Could you check a few things on this model? Use its own coordinates, in mm. A direction names the side the tool comes from. Coordinates: 2 decimals unless noted, no trailing zeros. Write each loop counter-clockwise with the first axis right and the second up, starting at its lowest first coordinate (ties: lowest second). Pieces come first, ordered by that corner, then holes. Notation, with made-up numbers: M 4.25,-16 L 45.25,-16 A10 ccw 45.25,-4 Z; hole C 30,47 d3. An arc over 180 degrees is marked long. Answer as CSV lines item,"result". Start each with the question number.
Item 1: If I drill on line 1 along Y through (x, z) = (52, 2.1); line 2 along Y through (x, z) = (54, 4.25); line 3 along Y through (x, z) = (6.5, 2), over which ranges is the centre line in solid material (lowest first)? Write a range as [from, to].
Item 2: Suppose I cut it at A-A, the plane y = 80. Write out the boundary of the cut face in (x, z).
Item 3: We'd pull the mould along X, two halves only. Please class faces 1 (the flat face through (30, 100, 10)), 2 (the cylindrical face through (29.133, 76.095, 10.274)), 3 (the cylindrical face through (49.253, 6.121, 8.549)), 4 (the flat face through (0, 42, 6)): +X half, -X half, draft (parallel to the pull), parting line (faces both ways), or undercut.
Item 4: I'm going to push flat-ended pins straight in: P1, Ø5, axis at x = 8.5, y = 6, coming from the -Z side; P2, Ø14, axis at x = 43, y = 80, coming from the -Z side; P3, Ø7, axis at x = 27.5, z = 4, coming from the +Y side. Where does each tip first touch, or does it pass through?
Item 5: Suppose I cut it at B-B, the plane x = 30. Write out the boundary of the cut face in (y, z), and give its area (3 significant figures).
Item 6: Suppose I cut it at D-D, the plane z = 1. Write out the boundary of the cut face in (x, y), and give its area (3 significant figures).
Item 7: On a 3-axis mill with a long thin cutter (end or side, diameter ignored), from which of +Z, -Z, +X, -X, +Y, -Y can I reach the whole of each face in a straight line? I mean faces 5 (the cylindrical face through (53.328, 68.054, 5.916)), 6 (the cylindrical face through (57, 6, 2)), 7 (the flat face through (30, 86, 8.5)). Say none if no direction works.
Item 8: Suppose I cut it at C-C, the plane y = 6. Write out the boundary of the cut face in (x, z).
```python
from build123d import *

# Parameters (mm, degrees)
ESQUISSE2_W                                        = 60
ESQUISSE2_H                                        = 100
BOSS_EXTRU_1_DEPTH                                 = 12
ESQUISSE3_R                                        = 4
ENL_V_MAT_EXTRU_1_DEPTH                            = 3.5
ESQUISSE5_W                                        = 8.5
ESQUISSE5_H                                        = 28
ENL_V_MAT_EXTRU_2_DEPTH                            = 61
TROU_TARAUD_M31_D                                  = 2.5
TROU_TARAUD_M32_D                                  = 2.5
CHAMBRAGE_POUR_VIS_T_TE_HEXAGONALE_M51_D           = 5.5
CHAMBRAGE_POUR_VIS_T_TE_HEXAGONALE_M51_CBORE_D     = 10
CHAMBRAGE_POUR_VIS_T_TE_HEXAGONALE_M51_CBORE_DEPTH = 5
CHAMBRAGE_POUR_VIS_T_TE_HEXAGONALE_M52_D           = 5.5
CHAMBRAGE_POUR_VIS_T_TE_HEXAGONALE_M52_CBORE_D     = 10
CHAMBRAGE_POUR_VIS_T_TE_HEXAGONALE_M52_CBORE_DEPTH = 5
CHANFREIN1_SIZE                                    = 15


with BuildPart() as part:
    # Esquisse2 → Boss.-Extru.1 (new body)
    with BuildSketch(Plane.XY):
        with Locations((30, 50)):
            Rectangle(ESQUISSE2_W, ESQUISSE2_H)
    extrude(amount=BOSS_EXTRU_1_DEPTH)

    # Esquisse3 → Enlèv. mat.-Extru.1 (cut)
    with BuildSketch(Plane.XY.offset(12)):
        with Locations((30, 80)):
            Circle(ESQUISSE3_R)
    extrude(amount=-ENL_V_MAT_EXTRU_1_DEPTH, mode=Mode.SUBTRACT)

    # Esquisse5 → Enlèv. mat.-Extru.2 (cut, through all)
    with BuildSketch(Plane.ZY):
        with Locations((4.25, 86)):
            Rectangle(ESQUISSE5_W, ESQUISSE5_H)
    extrude(amount=-ENL_V_MAT_EXTRU_2_DEPTH, mode=Mode.SUBTRACT)

    # Trou taraudé M31 (through all)
    with Locations(Plane.XY.offset(12)):
        with Locations((54, 67), (30, 80)):
            Hole(TROU_TARAUD_M31_D / 2)

    # Trou taraudé M32 (through all)
    with Locations(Plane.XY.offset(12)):
        with Locations((6, 67)):
            Hole(TROU_TARAUD_M32_D / 2)

    # Chambrage pour vis à tête hexagonale M51 (through all)
    with Locations(Plane(origin=(0, 0, 0), x_dir=(-1, 0, 0), z_dir=(0, 0, -1))):
        with Locations((-8, 6)):
            CounterBoreHole(CHAMBRAGE_POUR_VIS_T_TE_HEXAGONALE_M51_D / 2, CHAMBRAGE_POUR_VIS_T_TE_HEXAGONALE_M51_CBORE_D / 2, CHAMBRAGE_POUR_VIS_T_TE_HEXAGONALE_M51_CBORE_DEPTH)

    # Chambrage pour vis à tête hexagonale M52 (through all)
    with Locations(Plane(origin=(0, 0, 0), x_dir=(-1, 0, 0), z_dir=(0, 0, -1))):
        with Locations((-52, 6)):
            CounterBoreHole(CHAMBRAGE_POUR_VIS_T_TE_HEXAGONALE_M52_D / 2, CHAMBRAGE_POUR_VIS_T_TE_HEXAGONALE_M52_CBORE_D / 2, CHAMBRAGE_POUR_VIS_T_TE_HEXAGONALE_M52_CBORE_DEPTH)

    # Chanfrein1
    chanfrein1_edges = [part.edges().sort_by_distance(p)[0] for p in [
        (0, 100, 10.25),
        (60, 100, 10.25),
    ]]
    chamfer(chanfrein1_edges, length=CHANFREIN1_SIZE)


solid = part.part
```
Ans:
1,line 1,"y = [0, 1], [11, 72]"
1,line 2,"y = [0, 1.42], [10.58, 65.75], [68.25, 72]"
1,line 3,"y = [0, 1.23], [10.77, 65.85], [68.15, 72]"
2,outline,"M 0,8.5 L 26,8.5 L 26,12 L 0,12 Z; M 34,8.5 L 60,8.5 L 60,12 L 34,12 Z"
3,face 1,"draft"
3,face 2,"undercut"
3,face 3,"undercut"
3,face 4,"-X half"
4,P1,"stops at z = 5"
4,P2,"stops at z = 8.5"
4,P3,"stops at y = 72"
5,outline,"M 0,0 L 72,0 L 72,8.5 L 76,8.5 L 76,12 L 0,12 Z; M 84,8.5 L 100,8.5 L 100,12 L 84,12 Z"
5,area,"934 mm^2"
6,outline,"M 0,0 L 60,0 L 60,72 L 0,72 Z; hole C 8,6 d10; hole C 6,67 d2.5; hole C 52,6 d10; hole C 54,67 d2.5"
6,area,"4,150 mm^2"
7,face 5,"+Z, -Z"
7,face 6,"-Z"
7,face 7,"-Z, +X, -X, +Y"
8,outline,"M 0,0 L 3,0 L 3,5 L 5.25,5 L 5.25,12 L 0,12 Z; M 10.75,5 L 13,5 L 13,0 L 47,0 L 47,5 L 49.25,5 L 49.25,12 L 10.75,12 Z; M 54.75,5 L 57,5 L 57,0 L 60,0 L 60,12 L 54.75,12 Z"
